```python
from build123d import *

# Parameters (mm, degrees)
F0_W     = 76
F0_H     = 26
F1_DEPTH = 5
F2_W     = 90
F2_H     = 35
F3_DEPTH = 3
F4_R     = 5


with BuildPart() as f1:
    # F0 (on Front) → F1 (new body)
    with BuildSketch(Plane.XZ):
        Rectangle(F0_W, F0_H)
    extrude(amount=F1_DEPTH)

    # F2 (on face) → F3 (join)
    with BuildSketch(Plane.XZ.offset(5)):
        Rectangle(F2_W, F2_H)
    extrude(amount=F3_DEPTH)

    # F4
    f4_edges = [f1.edges().sort_by_distance(p)[0] for p in [
        (-38, -2.5, 13),
        (38, -2.5, 13),
        (38, -2.5, -13),
        (-38, -2.5, -13),
    ]]
    fillet(f4_edges, radius=F4_R)


solid = f1.part
```
Part model, mm, in its own coordinate system. A direction names the side the tool comes from. Give positions to 0.01 mm unless a question says otherwise; leave off trailing zeros. Write each loop counter-clockwise with the first axis right and the second up, starting at its lowest first coordinate (ties: lowest second). Pieces come first, ordered by that corner, then holes. Notation, with made-up numbers: (60, 73.5) -> (96, 73.5) arc R19 ccw to (96, 108.5) -> close; hole circle Ø11 at (-8.75, 33.25). An arc over 180 degrees is marked (long way). Put each result on its own line as item: value. Start each with the question number.
Item 1: Cut at A-A (x = 24). List the corners of the cut face in (y, z), then the cut area to 3 significant figures.
Item 2: Pin check, flat tips, straight feed: pin 1 Ø4 at (x, y) = (-9.5, -1.5) entering from +Z; pin 2 Ø4 at (x, y) = (-10.5, -2.5) entering from -Z; pin 3 Ø4 at (y, z) = (-2, -1) entering from -X. Stop position of each tip, or through.
Item 3: Which spindle directions (+Z, -Z, +X, -X, +Y, -Y) get a long thin tool onto all of the face, cutting with end or side? Do faces 1 (the face through (-1, -5, -15)), 2 (the face through (37, -3, 11)), 3 (the face through (-36, -3, -12)). Say none if no direction does.
Item 4: Cut at C-C (z = 14.5). List the corners of the cut face in (x, y), then the cut area to 3 significant figures.
Item 5: Wall check: L1, parallel to Z at x = -6, y = -2.25; L2, parallel to X at y = -4, z = -1; L3, parallel to Y at x = 4.5, z = -14. Give the ranges that are in metal, low to high. Write a range as [from, to].
Item 6: Cut at B-B (z = 0). List the corners of the cut face in (x, y), then the cut area to 3 significant figures.
Answer list:
1. outline: (-8, -17.5) -> (-5, -17.5) -> (-5, -13) -> (0, -13) -> (0, 13) -> (-5, 13) -> (-5, 17.5) -> (-8, 17.5) -> close
1. area: 235 mm2
2. pin 1: stops at z = 13
2. pin 2: stops at z = -13
2. pin 3: stops at x = -38
3. face 1: +Y
3. face 2: +Z, +X, +Y
3. face 3: -Z, -X, +Y
4. outline: (-45, -8) -> (45, -8) -> (45, -5) -> (-45, -5) -> close
4. area: 270 mm2
5. L1: z = [-13, 13]
5. L2: x = [-38, 38]
5. L3: y = [-8, -5]
6. outline: (-45, -8) -> (45, -8) -> (45, -5) -> (38, -5) -> (38, 0) -> (-38, 0) -> (-38, -5) -> (-45, -5) -> close
6. area: 650 mm2
